Build history of the part. All positions in model axes, mm. Face numbers are marked on the shaded views. A direction names the side the tool comes from. Round coordinates to 2 decimals unless told otherwise and drop trailing zeros. Write each loop counter-clockwise with the first axis right and the second up, starting at its lowest first coordinate (ties: lowest second). Pieces come first, ordered by that corner, then holes.
1) Pull direction Y, two halves, no side cores. Call the marked faces 1, 2, 3 and 4: +Y half, -Y half, draft (parallel to the pull), parting line (faces both ways), or undercut.
2) Saw through at C-C (x = 39.5). Write the cut outline in (y, z), plus the area to 3 significant figures.
3) Saw through at B-B (z = 115). Write the cut outline in (x, y).
4) Which spindle directions (+Z, -Z, +X, -X, +Y, -Y) get a long thin tool onto all of the face, cutting with end or side? Do the marked faces 5, 6 and 7. Say none if no direction does.
5) Saw through at A-A (y = 0). Write the cut outline in (x, z).
6) Saw through at D-D (x = 0). Write the cut outline in (y, z), plus the area to 3 significant figures.
7) Flat gauge pins, fed straight in: pin 1 (7.5 mm diameter, centred on x = 40.5, z = 104, fed in from +Y); pin 2 (2 mm diameter, centred on x = -15, z = 26.5, fed in from -Y); pin 3 (16.5 mm diameter, centred on x = -46, z = 92, fed in from -Y). Where does each tip first touch, or does it go through?
8) Wall check: probe 1 along X at (y, z) = (-13.5, 92); probe 2 along Y at (x, z) = (0, 14.5); probe 3 along Y at (x, z) = (-45.5, 115). Give the ranges that are in metal, low to high.
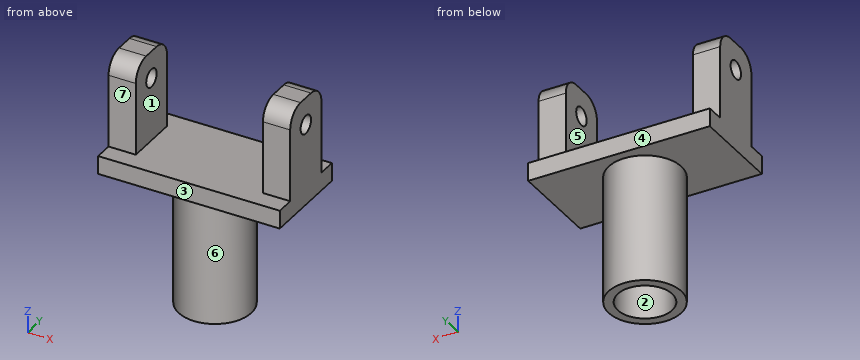
from build123d import *

# Parameters (mm, degrees)
SKETCH_1_R             = 20
SKETCH_1_R_2           = 15
EXTRUDE_1_DEPTH        = 70
SKETCH_2_W             = 100
SKETCH_2_H             = 50
EXTRUDE_2_DEPTH        = 10
SKETCH_3_W             = 15
SKETCH_3_H             = 30
EXTRUDE_3_DEPTH        = 50
FILLET_1_R             = 10
SKETCH_4_R             = 5
CUT_EXTRUDE_1_DEPTH    = 50
FILLET_1_OF_MIRROR_2_R = 10


with BuildPart() as part:
    # Эскиз1 → Бобышка-Вытянуть1 (new body)
    with BuildSketch(Plane.XY):
        Circle(SKETCH_1_R)
        Circle(SKETCH_1_R_2, mode=Mode.SUBTRACT)
    extrude(amount=EXTRUDE_1_DEPTH)

    # Эскиз2 → Бобышка-Вытянуть2 (add)
    with BuildSketch(Plane.XY.offset(70)):
        Rectangle(SKETCH_2_W, SKETCH_2_H)
    extrude(amount=EXTRUDE_2_DEPTH)

    # Эскиз3 → Бобышка-Вытянуть3 (add)
    with BuildSketch(Plane.XY.offset(80)):
        with Locations((-42.5, 0)):
            Rectangle(SKETCH_3_W, SKETCH_3_H)
    extrude_3 = extrude(amount=EXTRUDE_3_DEPTH)

    # Скругление1
    fillet_1_edges = [part.edges().sort_by_distance(p)[0] for p in [
        (-42.5, 15, 130),
        (-42.5, -15, 130),
    ]]
    fillet(fillet_1_edges, radius=FILLET_1_R)

    # Эскиз4 → Вырез-Вытянуть1 (cut)
    with BuildSketch(Plane.ZY.offset(50)):
        with Locations((115, 0)):
            Circle(SKETCH_4_R)
    cut_extrude_1 = extrude(amount=-CUT_EXTRUDE_1_DEPTH, mode=Mode.SUBTRACT)

    # Зеркальное отражение2: Бобышка-Вытянуть3, Вырез-Вытянуть1 across plane
    add(extrude_3.mirror(Plane(origin=(0, 0, 0), x_dir=(0, 0, 1), z_dir=(1, 0, 0))))
    add(cut_extrude_1.mirror(Plane(origin=(0, 0, 0), x_dir=(0, 0, 1), z_dir=(1, 0, 0))), mode=Mode.SUBTRACT)

    # Скругление1 of Зеркальное отражение2
    fillet_1_of_mirror_2_edges = [part.edges().sort_by_distance(p)[0] for p in [
        (42.5, 15, 130),
        (42.5, -15, 130),
    ]]
    fillet(fillet_1_of_mirror_2_edges, radius=FILLET_1_OF_MIRROR_2_R)


solid = part.part
Evaluation:
1. face 1: draft
1. face 2: undercut
1. face 3: -Y half
1. face 4: +Y half
2. outline: (-25, 70) - (25, 70) - (25, 80) - (15, 80) - (15, 120) arc R10 ccw to (5, 130) - (-5, 130) arc R10 ccw to (-15, 120) - (-15, 80) - (-25, 80) - close; hole circle Ø10 at (0, 115)
2. area: 1,880 mm2
3. outline: (-50, -15) - (-35, -15) - (-35, -5) - (-50, -5) - close; (-50, 5) - (-35, 5) - (-35, 15) - (-50, 15) - close; (35, -15) - (50, -15) - (50, -5) - (35, -5) - close; (35, 5) - (50, 5) - (50, 15) - (35, 15) - close
4. face 5: +Z, +Y, -Y
4. face 6: -Z
4. face 7: +Z, +X, -X, -Y
5. outline: (-50, 70) - (-20, 70) - (-20, 0) - (-15, 0) - (-15, 70) - (15, 70) - (15, 0) - (20, 0) - (20, 70) - (50, 70) - (50, 110) - (35, 110) - (35, 80) - (-35, 80) - (-35, 110) - (-50, 110) - close; (-50, 120) - (-35, 120) - (-35, 130) - (-50, 130) - close; (35, 120) - (50, 120) - (50, 130) - (35, 130) - close
6. outline: (-25, 70) - (-20, 70) - (-20, 0) - (-15, 0) - (-15, 70) - (15, 70) - (15, 0) - (20, 0) - (20, 70) - (25, 70) - (25, 80) - (-25, 80) - close
6. area: 1,200 mm2
7. pin 1: stops at y = 15
7. pin 2: stops at y = -14.28
7. pin 3: stops at y = -15
8. probe 1: x = -50 to -35, 35 to 50
8. probe 2: y = -20 to -15, 15 to 20
8. probe 3: y = -15 to -5, 5 to 15
